Part model, mm, in its own coordinate system. Face numbers are marked on the shaded views. A direction names the side the tool comes from. Coordinates: 2 decimals unless noted, no trailing zeros. Loops run counter-clockwise (first coordinate to the right, second up) from the corner with the lowest first, then second, coordinate; pieces in that order, holes last.
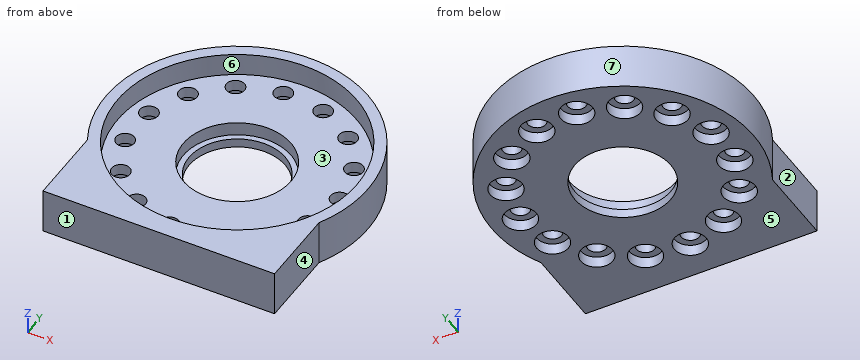
Autodesk Inventor part; units mm, degrees
ref_plane "YZ Plane" through (0, 0, 0) normal (1, 0, 0) x (0, 1, 0)
ref_plane "XZ Plane" through (0, 0, 0) normal (0, 1, 0) x (-1, 0, 0)
ref_plane "XY Plane" through (0, 0, 0) normal (0, 0, 1) x (1, 0, 0)
sketch "Sketch1" plane through (0, 0, 0) normal (0, 0, 1) x (1, 0, 0)
  circle A0 centre (0, 0) radius 45 construction
  circle A1 centre (45, 0) radius 4
  circle A2 centre (0, 0) radius 52.5
  circle A3 centre (0, 0) radius 57.5
  circle A4 centre (0, 0) radius 23.6
  circle A5 centre (0, 0) radius 21.1
  line L0 (50.8901, -26.7665) -> (50.8901, -61.7665)
  line L1 (50.8901, -61.7665) -> (-50.8901, -61.7665)
  line L2 (-50.8901, -61.7665) -> (-50.8901, -26.7665)
  line L3 (12, -56.7665) -> (-20, -56.7665) construction
  dimension "d0" = 90
  dimension "d1" = 8
  dimension "d2" = 105
  dimension "d3" = 5
  dimension "d16" = 47.2
  dimension "d20" = 2.5
  dimension "d27" = 35
  dimension "d28" = 5
extrude "Extrusion1" add sketch "Sketch1" along normal blind 20 contours A3 | A3 L0 L1 L2
extrude "Extrusion2" add sketch "Sketch1" along normal blind 10 contours A1 | A2
extrude "Extrusion3" cut sketch "Sketch1" along normal through all contours A1
pattern_circular "Circular Pattern2" count 15 over 360 about axis through (0, 0, -10) along (0, 0, 1) of "Extrusion3"
extrude "Extrusion4" add sketch "Sketch1" along normal blind 4 contours A4
sketch "Sketch2" plane through (0, 0, 0) normal (0, 0, -1) x (1, 0, 0)
  circle A0 centre (-44.0166, -9.356) radius 7
  circle A1 centre (-44.0166, -9.356) radius 4
  point P0 (0, 0)
  dimension "d21" = 14
extrude "Extrusion5" cut sketch "Sketch2" against normal blind 5
pattern_circular "Circular Pattern3" count 15 over 360 about axis through (0, 0, 0) along (0, 0, 1) of "Extrusion5"
properties part number "RearCover" material "Lead"
Q1. Tool access for the marked faces 1, 2, 3 and 4: list every direction of +Z, -Z, +X, -X, +Y, -Y with a clear straight run to the whole face (end or side of a thin tool).
Q2. Saw through at A-A (y = 0). List the corners of the cut face in (x, z).
Q3. Probe line 1 (X direction, y = -30, z = 7.5); line 2 (X direction, y = 37, z = 3); line 3 (Y direction, x = -45.5, z = 9). List the from-to ranges inside material, lowest first.
Q4. Mould opens along Y. For the marked faces 5, 6 and 7 say: released by +Y, released by -Y, zero draft, split by the parting line, or undercut.
Q5. Drop flat-ended pins along their axis: P1, Ø8.5, axis at x = 41.11, y = -18.3, coming from the -Z side; P2, Ø4, axis at x = -37, y = 27.5, coming from the -Z side; P3, Ø12.5, axis at x = -36.41, y = -26.45, coming from the +Z side; P4, Ø3, axis at x = 30, z = 6, coming from the +Y side. Give the stop position or say it passes through.
Q6. Saw through at B-B (z = 13.5). List the corners of the cut face in (x, y), plus the area to 3 significant figures.
Checked values:
1. face 1: +Z, -Z, +X, -X, -Y
1. face 2: +Z, -Z, -X, -Y
1. face 3: +Z
1. face 4: +Z, -Z, +X, -Y
2. outline: (-57.5, 0) - (-21.1, 0) - (-21.1, 4) - (-23.6, 4) - (-23.6, 10) - (-52.5, 10) - (-52.5, 20) - (-57.5, 20) - close; (21.1, 0) - (38, 0) - (38, 5) - (41, 5) - (41, 10) - (23.6, 10) - (23.6, 4) - (21.1, 4) - close; (49, 5) - (52, 5) - (52, 0) - (57.5, 0) - (57.5, 20) - (52.5, 20) - (52.5, 10) - (49, 10) - close
3. line 1: x = -50.89 to -38.25, -34.56 to 28.07, 32.15 to 50.89
3. line 2: x = -44.01 to -29.22, -15.78 to 9.98, 17.83 to 24.08, 36.14 to 44.01
3. line 3: y = -61.77 to -13.07, -5.64 to 5.64, 13.07 to 35.16
4. face 5: zero draft
4. face 6: undercut
4. face 7: split by the parting line
5. P1: stops at z = 5
5. P2: passes through
5. P3: stops at z = 10
5. P4: stops at y = 49.94
6. outline: (-50.89, -61.77) - (50.89, -61.77) - (50.89, -26.77) arc R57.5 ccw (long way) to (-50.89, -26.77) - close; hole circle Ø105 at (0, 0)
6. area: 3,060 mm2
